from build123d import *

# Parameters (mm, degrees)
EXTRUDE_1_DEPTH     = 80
CUT_EXTRUDE_1_DEPTH = 338.16811987
CUT_EXTRUDE_4_DEPTH = 258.724089853
EXTRUDE_2_DEPTH     = 236
SKETCH_8_W          = 29
SKETCH_8_H          = 45.03
CUT_EXTRUDE_5_DEPTH = 333.864316987
SKETCH_11_W         = 1.5
SKETCH_11_H         = 2.5
SKETCH_12_R         = 1.5
CUT_EXTRUDE_6_DEPTH = 53


with BuildPart() as part:
    # Эскиз1 → Бобышка-Вытянуть1 (new body)
    with BuildSketch(Plane(origin=(0, 0, 0), x_dir=(0, 0, -1), z_dir=(1, 0, 0))):
        with BuildLine():
            Line((0, 0), (0, 324))
            Line((0, 324), (51, 324))
            Line((51, 324), (47.202681995, 251.542856107))
            ThreePointArc((47.202681995, 251.542856107), (38.415146245, 245.880357077), (35, 236))
            Line((35, 236), (22, 236))
            Line((22, 236), (22, 0))
            Line((22, 0), (0, 0))
        make_face()
    extrude(amount=-EXTRUDE_1_DEPTH)

    # Вырез-По сечениям1: read off the stored shape, not the designer's step
    # Вырез-По сечениям1: loft between two sections, ruled curve by curve
    loft_1_from = [
        Edge.make_bspline([(-39.686086493, 386.998880194, -51), (-41.519373167, 387.011959923, -51), (-43.469191145, 386.912155262, -51), (-47.589656467, 386.390203752, -51), (-49.760899046, 385.967798341, -51), (-54.275759928, 384.685843196, -51), (-56.619984777, 383.82558407, -51), (-61.376492683, 381.5486416, -51), (-63.789033826, 380.130665414, -51), (-68.507360794, 376.644239105, -51), (-70.812489477, 374.574106824, -51), (-74.008903802, 370.963867661, -51), (-75.030367598, 369.677012554, -51), (-76.951946734, 366.944587811, -51), (-77.851980564, 365.498997396, -51), (-79.497654124, 362.465678388, -51), (-80.243201605, 360.877958795, -51), (-81.549913197, 357.585657318, -51), (-82.110987295, 355.881119395, -51), (-83.024607662, 352.388377038, -51), (-83.377081555, 350.600250078, -51), (-83.857698345, 346.979610705, -51), (-83.985800464, 345.147200182, -51), (-84.011959923, 341.480626833, -51), (-83.910016471, 339.646575032, -51), (-83.481109456, 336.019446589, -51), (-83.154185214, 334.226472409, -51), (-82.290493812, 330.721049679, -51), (-81.753797915, 329.008679629, -51), (-80.494195327, 325.69806858, -51), (-79.771378013, 324.099872821, -51), (-78.169152689, 321.043381421, -51), (-77.289836791, 319.585096094, -51), (-75.407440689, 316.825531587, -51), (-74.404442283, 315.524232794, -51), (-71.259865805, 311.868753328, -51), (-68.984509326, 309.765941211, -51), (-64.316408519, 306.212546688, -51), (-61.924345268, 304.76029167, -51), (-57.200809972, 302.415713078, -51), (-54.869098312, 301.522093112, -51), (-50.372988531, 300.17584848, -51), (-48.207994046, 299.722505841, -51), (-44.095395614, 299.141814883, -51), (-42.147200182, 299.014199536, -51), (-38.480626833, 298.988040077, -51), (-36.530808855, 299.087844738, -51), (-32.410343533, 299.609796248, -51), (-30.239100954, 300.032201659, -51), (-25.724240072, 301.314156804, -51), (-23.380015223, 302.17441593, -51), (-18.623507317, 304.4513584, -51), (-16.210966174, 305.869334586, -51), (-11.492639206, 309.355760895, -51), (-9.187510523, 311.425893176, -51), (-5.991096198, 315.036132339, -51), (-4.969632402, 316.322987446, -51), (-3.048053266, 319.055412189, -51), (-2.148019436, 320.501002604, -51), (-0.502345876, 323.534321612, -51), (0.243201605, 325.122041205, -51), (1.549913197, 328.414342682, -51), (2.110987295, 330.118880605, -51), (3.024607662, 333.611622962, -51), (3.377081555, 335.399749922, -51), (3.857698345, 339.020389295, -51), (3.985800464, 340.852799818, -51), (4.011959923, 344.519373167, -51), (3.910016471, 346.353424968, -51), (3.481109456, 349.980553411, -51), (3.154185214, 351.773527591, -51), (2.290493812, 355.278950321, -51), (1.753797915, 356.991320371, -51), (0.494195327, 360.30193142, -51), (-0.228621987, 361.900127179, -51), (-1.830847311, 364.956618579, -51), (-2.710163209, 366.414903906, -51), (-4.592559311, 369.174468413, -51), (-5.595557717, 370.475767206, -51), (-8.740134195, 374.131246672, -51), (-11.015490674, 376.234058789, -51), (-15.683591481, 379.787453312, -51), (-18.075654732, 381.23970833, -51), (-22.799190028, 383.584286922, -51), (-25.130901688, 384.477906888, -51), (-29.627011469, 385.82415152, -51), (-31.792005954, 386.277494159, -51), (-35.904604386, 386.858185117, -51), (-37.852799818, 386.985800464, -51), (-39.686086493, 386.998880194, -51)], [0.5, 0.5, 0.5, 0.5, 0.53125, 0.53125, 0.5625, 0.5625, 0.59375, 0.59375, 0.625, 0.625, 0.65625, 0.65625, 0.671875, 0.671875, 0.6875, 0.6875, 0.703125, 0.703125, 0.71875, 0.71875, 0.734375, 0.734375, 0.75, 0.75, 0.765625, 0.765625, 0.78125, 0.78125, 0.796875, 0.796875, 0.8125, 0.8125, 0.828125, 0.828125, 0.84375, 0.84375, 0.875, 0.875, 0.90625, 0.90625, 0.9375, 0.9375, 0.96875, 0.96875, 1, 1, 1.03125, 1.03125, 1.0625, 1.0625, 1.09375, 1.09375, 1.125, 1.125, 1.15625, 1.15625, 1.171875, 1.171875, 1.1875, 1.1875, 1.203125, 1.203125, 1.21875, 1.21875, 1.234375, 1.234375, 1.25, 1.25, 1.265625, 1.265625, 1.28125, 1.28125, 1.296875, 1.296875, 1.3125, 1.3125, 1.328125, 1.328125, 1.34375, 1.34375, 1.375, 1.375, 1.40625, 1.40625, 1.4375, 1.4375, 1.46875, 1.46875, 1.5, 1.5, 1.5, 1.5], 3),
    ]
    loft_1_to = [
        Edge.make_bspline([(-40.713360954, 406.994910903, 0), (-42.796482241, 406.965187529, 0), (-45.009249926, 406.804381918, 0), (-49.677831319, 406.111186343, 0), (-52.134314987, 405.57848815, 0), (-57.232488149, 404.012258649, 0), (-59.874849492, 402.977906649, 0), (-65.223361777, 400.275392116, 0), (-67.929774494, 398.605754504, 0), (-73.205496114, 394.530069796, 0), (-75.774017529, 392.122127574, 0), (-79.317678059, 387.942789724, 0), (-80.446871791, 386.455948521, 0), (-82.56353512, 383.304901046, 0), (-83.550911607, 381.64067315, 0), (-85.346800294, 378.15448837, 0), (-86.155207908, 376.332543952, 0), (-87.559702616, 372.560371453, 0), (-88.155688516, 370.610195503, 0), (-89.108716472, 366.619860939, 0), (-89.465678189, 364.579792104, 0), (-89.923659015, 360.454683427, 0), (-90.024634276, 358.369760334, 0), (-89.965187529, 354.203517759, 0), (-89.804767323, 352.122324432, 0), (-89.229277266, 348.011962011, 0), (-88.814254578, 345.982908368, 0), (-87.74776424, 342.021389647, 0), (-87.09637946, 340.08901202, 0), (-85.584830664, 336.358447587, 0), (-84.72476929, 334.560310005, 0), (-82.830145523, 331.126783934, 0), (-81.795688029, 329.491404922, 0), (-79.589982191, 326.402031913, 0), (-78.418826302, 324.948013642, 0), (-74.757365501, 320.871483301, 0), (-72.121187465, 318.537805224, 0), (-66.731328092, 314.614304187, 0), (-63.978379853, 313.022564402, 0), (-58.5549381, 310.473751342, 0), (-55.884140832, 309.515211055, 0), (-50.743356242, 308.095077878, 0), (-48.27267393, 307.632683797, 0), (-43.586215216, 307.072972214, 0), (-41.369760334, 306.975365724, 0), (-37.203517759, 307.034812471, 0), (-34.990750074, 307.195618082, 0), (-30.322168681, 307.888813657, 0), (-27.865685013, 308.42151185, 0), (-22.767511851, 309.987741351, 0), (-20.125150508, 311.022093351, 0), (-14.776638223, 313.724607884, 0), (-12.070225506, 315.394245496, 0), (-6.794503886, 319.469930204, 0), (-4.225982471, 321.877872426, 0), (-0.682321941, 326.057210276, 0), (0.446871791, 327.544051479, 0), (2.56353512, 330.695098954, 0), (3.550911607, 332.35932685, 0), (5.346800294, 335.84551163, 0), (6.155207908, 337.667456048, 0), (7.559702616, 341.439628547, 0), (8.155688516, 343.389804497, 0), (9.108716472, 347.380139061, 0), (9.465678189, 349.420207896, 0), (9.923659015, 353.545316573, 0), (10.024634276, 355.630239666, 0), (9.965187529, 359.796482241, 0), (9.804767323, 361.877675568, 0), (9.229277266, 365.988037989, 0), (8.814254578, 368.017091632, 0), (7.74776424, 371.978610353, 0), (7.09637946, 373.91098798, 0), (5.584830664, 377.641552413, 0), (4.72476929, 379.439689995, 0), (2.830145523, 382.873216066, 0), (1.795688029, 384.508595078, 0), (-0.410017809, 387.597968087, 0), (-1.581173698, 389.051986358, 0), (-5.242634499, 393.128516699, 0), (-7.878812535, 395.462194776, 0), (-13.268671908, 399.385695813, 0), (-16.021620147, 400.977435598, 0), (-21.4450619, 403.526248658, 0), (-24.115859168, 404.484788945, 0), (-29.256643758, 405.904922122, 0), (-31.72732607, 406.367316203, 0), (-36.413784784, 406.927027786, 0), (-38.630239666, 407.024634276, 0), (-40.713360954, 406.994910903, 0)], [0.5, 0.5, 0.5, 0.5, 0.53125, 0.53125, 0.5625, 0.5625, 0.59375, 0.59375, 0.625, 0.625, 0.65625, 0.65625, 0.671875, 0.671875, 0.6875, 0.6875, 0.703125, 0.703125, 0.71875, 0.71875, 0.734375, 0.734375, 0.75, 0.75, 0.765625, 0.765625, 0.78125, 0.78125, 0.796875, 0.796875, 0.8125, 0.8125, 0.828125, 0.828125, 0.84375, 0.84375, 0.875, 0.875, 0.90625, 0.90625, 0.9375, 0.9375, 0.96875, 0.96875, 1, 1, 1.03125, 1.03125, 1.0625, 1.0625, 1.09375, 1.09375, 1.125, 1.125, 1.15625, 1.15625, 1.171875, 1.171875, 1.1875, 1.1875, 1.203125, 1.203125, 1.21875, 1.21875, 1.234375, 1.234375, 1.25, 1.25, 1.265625, 1.265625, 1.28125, 1.28125, 1.296875, 1.296875, 1.3125, 1.3125, 1.328125, 1.328125, 1.34375, 1.34375, 1.375, 1.375, 1.40625, 1.40625, 1.4375, 1.4375, 1.46875, 1.46875, 1.5, 1.5, 1.5, 1.5], 3),
    ]
    loft_1 = Solid(Shell([*[Face.make_surface_from_curves(loft_1_from[k], loft_1_to[k]) for k in range(1)], Face(Wire(loft_1_from)), Face(Wire(loft_1_to))]))
    add(loft_1, mode=Mode.SUBTRACT)

    # Эскиз5 → Вырез-Вытянуть1 (cut, through all)
    with BuildSketch(Plane(origin=(0, -1.778022863, -33.926697283), x_dir=(-1, 0, 0), z_dir=(0, -0.05233595624294387, -0.998629534754574))):
        Polygon((80, 313.151391037), (56.299680313, 331.010862926), (80, 331.010862926), align=None)
        Polygon((0, 313.151391037), (23.700319687, 331.010862926), (0, 331.010862926), align=None)
    extrude(amount=-CUT_EXTRUDE_1_DEPTH, mode=Mode.SUBTRACT)

    # Эскиз3 → Вырез-Вытянуть4 (cut, through all)
    with BuildSketch(Plane(origin=(-50, 250.794151495, -32), x_dir=(-0.9397934234884354, -0.341743063086709, -1.1856594285774567e-15), z_dir=(0, 0, -1))):
        Polygon((0, 0), (20.675455317, 7.518347388), (23.409399821, 0), (2.733944505, -7.518347388), align=None)
    cut_extrude_4 = extrude(amount=CUT_EXTRUDE_4_DEPTH, mode=Mode.SUBTRACT)

    # Зеркальное отражение1: Вырез-Вытянуть4 across plane
    add(cut_extrude_4.mirror(Plane(origin=(-40, 0, 0), x_dir=(0, 0, 1), z_dir=(1, 0, 0))), mode=Mode.SUBTRACT)

    # Эскиз6 → Бобышка-Вытянуть2 (add)
    with BuildSketch(Plane.XZ.offset(-236)):
        Polygon((0, -22), (-40, -29), (-80, -22), align=None)
    extrude(amount=EXTRUDE_2_DEPTH)

    # Вырез-По траектории1: sweep along a curve in space
    with BuildLine() as sweep_1_path:
        Line((-40, 236, 0), (-40, 206.49134077, -49.110656108))
    # Эскиз8 → Вырез-По траектории1 (sweep, cut)
    with BuildSketch(Plane.XY):
        with Locations((-40, 213.485)):
            Rectangle(SKETCH_8_W, SKETCH_8_H)
    sweep(path=sweep_1_path.line, mode=Mode.SUBTRACT)

    # Эскиз9 → Вырез-Вытянуть5 (cut, through all)
    with BuildSketch(Plane.XY):
        Polygon((-54.5, 190.97), (-25.5, 190.97), (-25.5, 105.5), (-29, 102), (-29, 0), (-51, 0), (-51, 102), (-54.5, 105.5), align=None)
    extrude(amount=-CUT_EXTRUDE_5_DEPTH, mode=Mode.SUBTRACT)

    # Вырез-По траектории4: sweep along a curve in space
    with BuildLine() as sweep_4_path:
        Line((0, 62.25, 0), (0, 62.25, -22))
        Line((0, 62.25, -22), (-29, 62.25, -27.075))
    # Эскиз11 → Вырез-По траектории4 (sweep, cut)
    with BuildSketch(Plane.XY):
        with Locations((-0.75, 62.25)):
            Rectangle(SKETCH_11_W, SKETCH_11_H)
    sweep_4 = sweep(path=sweep_4_path.line, transition=Transition.RIGHT, mode=Mode.SUBTRACT)

    # Зеркальное отражение2: Вырез-По траектории4 across plane
    add(sweep_4.mirror(Plane(origin=(-40, 0, 0), x_dir=(0, 0, 1), z_dir=(1, 0, 0))), mode=Mode.SUBTRACT)

    # Эскиз12 → Вырез-Вытянуть6 (cut)
    with BuildSketch(Plane.XZ):
        with Locations((-20, -25.5)):
            Circle(SKETCH_12_R)
        with Locations((-9, -23.575)):
            Circle(SKETCH_12_R)
        with Locations((-60, -25.5)):
            Circle(SKETCH_12_R)
        with Locations((-71, -23.575)):
            Circle(SKETCH_12_R)
    extrude(amount=-CUT_EXTRUDE_6_DEPTH, mode=Mode.SUBTRACT)


solid = part.part
Could you check a few things on this model? Use its own coordinates, in mm. A direction names the side the tool comes from. Coordinates: 2 decimals unless noted, no trailing zeros. Order: outer loops, then holes, each group sorted by start corner. A loop starts at its lowest first (then second) coordinate and runs counter-clockwise, first axis right, second up.
Q1. Will these pins go through, and if not, where does the flat tip stop? pin 1 (2.5 mm diameter, centred on y = 245.5, z = -40, fed in from +X); pin 2 (1 mm diameter, centred on x = -13.5, z = -26.5, fed in from -Y); pin 3 (0.9 mm diameter, centred on x = -71, z = -23, fed in from -Y); pin 4 (2 mm diameter, centred on x = -57.5, y = 93.5, fed in from -Z).
Q2. Please list where these lines run through material, in increasing order: L1, parallel to X at y = 160, z = -9; L2, parallel to X at y = 20, z = -11; L3, parallel to Z at x = -69.5, y = 111.5.
Q3. Thinking about a two-plate mould opening in Y: for faces 5 (the flat face through (-61, 250.794, -38)), 6 (the flat face through (-71.9, 61, -22.1)), 7 (the flat face through (-14, 0, -13)), 8 (the flat face through (-51, 50, -13)), which applies, released by +Y, released by -Y, zero draft, split by the parting line, or undercut?
Q4. Suppose I cut it at A-A on y = 123. Please give me the cut outline in (x, z), and give its area (3 significant figures).
Q5. Which directions (+Z, -Z, +X, -X, +Y, -Y) give clear straight access to the entire face, cutting with the end or side of a thin tool? Please do faces 1 (the flat face through (-8.1, 63.5, -22.2)), 2 (the flat face through (-19, 250.794, -38)), 3 (the flat face through (-71.9, 63.5, -22.2)), 4 (the flat face through (-39.797, 227.166, -14.703)).
Q6. Suppose I cut it at C-C on y = 293. Please give me the cut outline in (x, z).
Q7. Suppose I cut it at B-B on y = 35. Please give me the cut outline in (x, z) (3 decimals).
Answer:
1. pin 1: passes through
1. pin 2: stops at y = 236
1. pin 3: stops at y = 53
1. pin 4: stops at z = -26.11
2. L1: x = -80 to -54.5, -25.5 to 0
2. L2: x = -80 to -51, -29 to 0
2. L3: z = -23.84 to 0
3. face 5: undercut
3. face 6: undercut
3. face 7: released by -Y
3. face 8: zero draft
4. outline: (-80, -22) - (-54.5, -26.46) - (-54.5, 0) - (-80, 0) - close; (-25.5, -26.46) - (0, -22) - (0, 0) - (-25.5, 0) - close
4. area: 1,240 mm2
5. face 1: -Z, +X
5. face 2: -Z
5. face 3: -Z, -X
5. face 4: +Z
6. outline: (-80, -49.38) - (0, -49.38) - (0, 0) - (-80, 0) - close
7. outline: (-80, -22) - (-72.478, -23.316) arc R1.5 cw to (-69.522, -23.834) - (-61.478, -25.241) arc R1.5 cw to (-58.522, -25.759) - (-51, -27.075) - (-51, 0) - (-80, 0) - close; (-29, -27.075) - (-21.478, -25.759) arc R1.5 cw to (-18.522, -25.241) - (-10.478, -23.834) arc R1.5 cw to (-7.522, -23.316) - (0, -22) - (0, 0) - (-29, 0) - close
